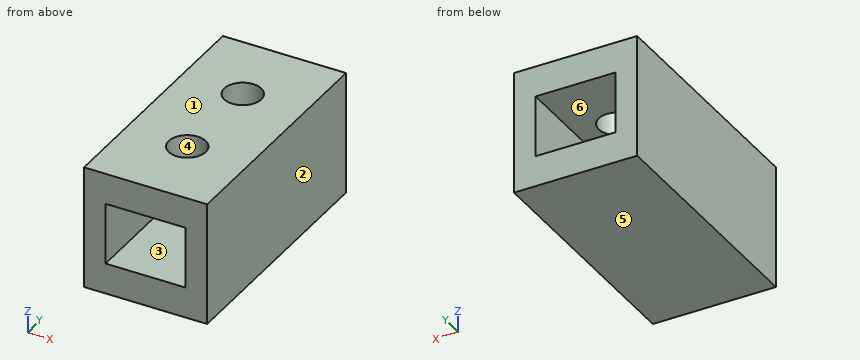
```python
from build123d import *

# Parameters (mm, degrees)
F0_W     = 25.4
F0_H     = 50.8
F1_DEPTH = 25.4
F2_W     = 16.51
F2_H     = 12.7
F3_DEPTH = 50.8
F4_R     = 3.81
F5_DEPTH = 15.24


with BuildPart() as f1:
    # F0 (on Top) → F1 (new body)
    with BuildSketch(Plane.XY):
        with Locations((2.239326, 0)):
            Rectangle(F0_W, F0_H)
    extrude(amount=F1_DEPTH)

    # F2 (on face) → F3 (cut)
    with BuildSketch(Plane.XZ.offset(25.4)):
        with Locations((2.239326, 12.7)):
            Rectangle(F2_W, F2_H)
    extrude(amount=-F3_DEPTH, mode=Mode.SUBTRACT)

    # F4 (on face) → F5 (cut)
    with BuildSketch(Plane.XY.offset(25.4)):
        with Locations((2.239326, 10.16)):
            Circle(F4_R)
        with Locations((2.239326, -10.16)):
            Circle(F4_R)
    extrude(amount=-F5_DEPTH, mode=Mode.SUBTRACT)


solid = f1.part
```
Verification items for the finished model (mm, model axes). Face numbers are marked on the shaded views. A direction names the side the tool comes from. Give positions to 0.01 mm unless a question says otherwise; leave off trailing zeros. Order: outer loops, then holes, each group sorted by start corner. A loop starts at its lowest first (then second) coordinate and runs counter-clockwise, first axis right, second up. Notation, with made-up numbers: (27, 56) - (75, 56) arc R32 ccw to (75, 89) - close; hole circle Ø1 at (5, 43). An arc over 180 degrees is marked (long way). Answer as CSV lines item,"result". Start each with the question number.
Item 1: Section check B-B, the plane x = -5.25. Record the boundary of the cut face in (y, z), plus the area to 3 significant figures.
Item 2: Section check D-D, the plane z = 22.25. Record the boundary of the cut face in (x, y).
Item 3: Mould release check, pull along Z, two halves, no side actions. Record for the marked faces 1, 2 and 3: released by +Z, released by -Z, zero draft, split by the parting line, or undercut.
Item 4: Gauge pin test, flat end, axial feed: pin 1 (5 mm diameter, centred on x = 2.5, y = 8, fed in from -Z). Record the tip position at first contact, or that the pin passes through.
Item 5: Access from +Z, -Z, +X, -X, +Y, -Y to the whole of each face (thin tool, end or side, straight path). Record for the marked faces 4, 5 and 6.
Item 6: Section check A-A, the plane z = 14. Record the boundary of the cut face in (x, y).
Item 7: Section check C-C, the plane y = -19. Record the boundary of the cut face in (x, z), plus the area to 3 significant figures.
Item 8: Material ranges on L1, parallel to X at y = 3, z = 9.5; L2, parallel to Z at x = -3.25, y = 8; L3, parallel to X at y = -8, z = 20.5, recorded low to high.
Filled in:
1,outline,"(-25.4, 0) - (25.4, 0) - (25.4, 6.35) - (-25.4, 6.35) - close; (-25.4, 19.05) - (25.4, 19.05) - (25.4, 25.4) - (-25.4, 25.4) - close"
1,area,"645 mm^2"
2,outline,"(-10.46, -25.4) - (14.94, -25.4) - (14.94, 25.4) - (-10.46, 25.4) - close; hole circle Ø7.62 at (2.24, -10.16); hole circle Ø7.62 at (2.24, 10.16)"
3,face 1,"released by +Z"
3,face 2,"zero draft"
3,face 3,"undercut"
4,pin 1,"z = 0"
5,face 4,"+Z"
5,face 5,"-Z, +X, -X, +Y, -Y"
5,face 6,"+Y, -Y"
6,outline,"(-10.46, -25.4) - (-6.02, -25.4) - (-6.02, 25.4) - (-10.46, 25.4) - close; (10.49, -25.4) - (14.94, -25.4) - (14.94, 25.4) - (10.49, 25.4) - close"
7,outline,"(-10.46, 0) - (14.94, 0) - (14.94, 25.4) - (-10.46, 25.4) - close; hole (-6.02, 6.35) - (10.49, 6.35) - (10.49, 19.05) - (-6.02, 19.05) - close"
7,area,"435 mm^2"
8,L1,"-10.46 to -6.02, 10.49 to 14.94"
8,L2,"0 to 6.35, 19.05 to 25.4"
8,L3,"-10.46 to -0.9, 5.38 to 14.94"
